Autodesk Inventor part; units mm, degrees
ref_plane "Plan YZ" through (0, 0, 0) normal (1, 0, 0) x (0, 1, 0)
ref_plane "Plan XZ" through (0, 0, 0) normal (0, 1, 0) x (-1, 0, 0)
ref_plane "Plan XY" through (0, 0, 0) normal (0, 0, 1) x (1, 0, 0)
sketch "Esquisse1" plane through (0, 0, 0) normal (0, 0, 1) x (1, 0, 0)
  line L0 (0, 0) -> (43.25, 0)
  line L1 (43.25, 0) -> (43.25, 42)
  line L2 (43.25, 42) -> (0, 42)
  line L3 (0, 42) -> (0, 0)
  dimension "d0" = 43.25
  dimension "d1" = 42
extrude "Extrusion1" add sketch "Esquisse1" along normal blind 1.6
sketch "Esquisse6" plane through (0, 0, 1.6) normal (0, 0, 1) x (1, 0, 0)
  line L0 (4.625, 38) -> (38.625, 38)
  line L1 (38.625, 38) -> (38.625, 4)
  line L2 (38.625, 4) -> (4.625, 4)
  line L3 (4.625, 4) -> (4.625, 38)
  line L4 (0, 27.3284) -> (4.625, 27.3284) construction
  line L5 (43.25, 21) -> (38.625, 21) construction
  line L6 (19.4191, 4) -> (19.4191, 0) construction
  line L7 (15.7943, 42) -> (15.7943, 38) construction
  line L8 (0, 0) -> (43.25, 0) construction
  line L9 (43.25, 42) -> (0, 42) construction
  line L10 (43.25, 0) -> (43.25, 42) construction
  line L11 (0, 42) -> (0, 0) construction
  dimension "d4" = 34
  dimension "d5" = 34
extrude "Extrusion2" add sketch "Esquisse6" along normal blind 1.9
sketch "Esquisse7" plane through (0, 0, 1.6) normal (0, 0, 1) x (1, 0, 0)
  line L0 (43.25, 0) -> (43.25, 42)
  line L1 (43.25, 42) -> (0, 42)
  point P0 (0, 0)
  point P1 (40.71, 39.46)
  dimension "d21" = 2.54
  dimension "d22" = 2.54
hole "Perçage1" at (40.71, 39.46, 1.6) direction (0, 0, -1) diameter 2.7 end through all
pattern_linear "Réseau rectangulaire1" count 2 spacing 36.9 along (0, -1, 0) count 2 spacing 38.1 along (-1, 0, 0) of "Perçage1"
sketch "Esquisse8" plane through (0, 0, 3.5) normal (0, 0, 1) x (1, 0, 0)
  line L0 (11.625, 24) -> (11.625, 19)
  line L1 (11.625, 19) -> (14.625, 19)
  line L2 (14.625, 19) -> (14.625, 20)
  line L3 (14.625, 20) -> (12.625, 20)
  line L4 (12.625, 20) -> (12.625, 24)
  line L5 (12.625, 24) -> (11.625, 24)
  line L6 (17.625, 24) -> (17.625, 19)
  line L7 (17.625, 19) -> (20.625, 19)
  line L8 (20.625, 19) -> (20.625, 20)
  line L9 (20.625, 20) -> (18.625, 20)
  line L10 (18.625, 20) -> (18.625, 21)
  line L11 (18.625, 21) -> (20.625, 21)
  line L12 (20.625, 21) -> (20.625, 22)
  line L13 (20.625, 22) -> (18.625, 22)
  line L14 (18.625, 22) -> (18.625, 23)
  line L15 (20.625, 23) -> (20.625, 24)
  line L16 (20.625, 24) -> (17.625, 24)
  line L17 (17.625, 24) -> (17.625, 24)
  line L18 (18.625, 23) -> (20.625, 23)
  line L19 (23.625, 19) -> (23.625, 24)
  line L20 (23.625, 24) -> (26.125, 24)
  line L21 (26.125, 24) -> (28.625, 21.5)
  line L22 (28.625, 21.5) -> (26.125, 19)
  line L23 (26.125, 19) -> (23.625, 19)
  line L24 (24.625, 20) -> (24.625, 23)
  line L25 (4.625, 38) -> (4.625, 4)
  line L26 (4.625, 4) -> (38.625, 4)
  line L27 (24.625, 20) -> (26.125, 20)
  line L28 (26.125, 20) -> (27.625, 21.5)
  line L29 (24.625, 23) -> (26.125, 23)
  line L30 (26.125, 23) -> (27.625, 21.5)
  point P0 (0, 0)
  dimension "d23" = 5
  dimension "d24" = 4
  dimension "d25" = 1
  dimension "d26" = 7
  dimension "d27" = 3
  dimension "d28" = 3
  dimension "d29" = 3
  dimension "d30" = 3
  dimension "d31" = 15
  dimension "d32" = 5
  dimension "d33" = 1
  dimension "d34" = 1
  dimension "d35" = 1
  dimension "d36" = 1
  dimension "d37" = 2
  dimension "d38" = 1
  dimension "d39" = 1
  dimension "d40" = 1
  dimension "d41" = 45
  dimension "d42" = 45
  dimension "d43" = 1
  dimension "d45" = 5
extrude "Extrusion3" cut sketch "Esquisse8" against normal blind 1
fillet "Congé1" radius 2 4 edges at (0, 42, 0.8) (43.25, 42, 0.8) (43.25, 0, 0.8) (0, 0, 0.8)
properties part number "P1704_014_Display" material "."
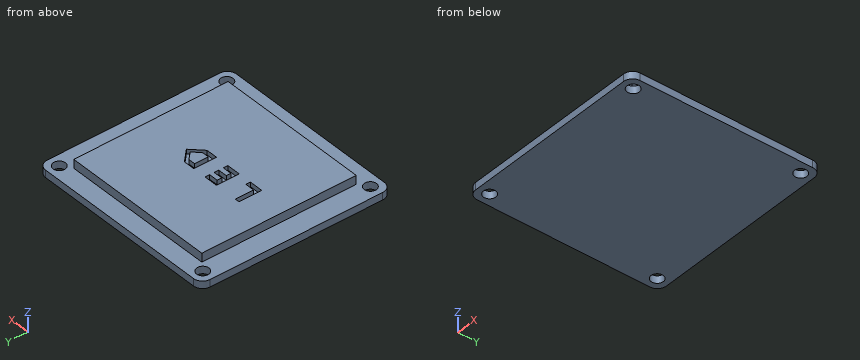
Source: CAD feature listing. Evaluate the final solid. Frame: model axes, mm. Round coordinates to 2 decimals unless told otherwise and drop trailing zeros. Order: outer loops, then holes, each group sorted by start corner. A loop starts at its lowest first (then second) coordinate and runs counter-clockwise, first axis right, second up. Notation, with made-up numbers: (0.5, 52.25) -> (32.5, 52.25) arc R16 cw to (32.5, 80.25) -> close; hole circle Ø1 at (86, 85.5). An arc over 180 degrees is marked (long way). One line per item, written item: value. Start each with the question number.
Q1. Material intervals for probe 1 along Y at (x, z) = (40.71, 1.05); probe 2 along X at (y, z) = (39.46, 1.25); probe 3 along Y at (x, z) = (18, 3.3), sorted ascending.
Q2. Pin query (flat end, axial travel): pin 1 (1.1 mm diameter, centred on x = 12, z = 3, fed in from -Y); pin 2 (1.1 mm diameter, centred on x = 19.5, z = 3, fed in from +Y); pin 3 (2.5 mm diameter, centred on x = 40.71, y = 2.56, fed in from -Z); pin 4 (1.1 mm diameter, centred on y = 21.5, z = 3, fed in from -X) (3 decimals). Return the tip coordinate at first contact, or that it passes through.
Q3. Section query C-C (x = 8). Return the cut outline in (y, z).
Q4. Section query B-B (y = 39.46). Return the cut outline in (x, z), plus the area to 3 significant figures.
Q5. Section query A-A (x = 2.61). Return the cut outline in (y, z), plus the area to 3 significant figures.
Q6. Section query D-D (y = 32.5). Return the cut outline in (x, z) (3 decimals), plus the area to 3 significant figures.
Findings below:
1. probe 1: 0 to 1.21, 3.91 to 38.11, 40.81 to 42
1. probe 2: 0 to 1.26, 3.96 to 39.36, 42.06 to 43.25
1. probe 3: 4 to 19, 24 to 38
2. pin 1: y = 4
2. pin 2: y = 38
2. pin 3: through
2. pin 4: x = 4.625
3. outline: (0, 0) -> (42, 0) -> (42, 1.6) -> (38, 1.6) -> (38, 3.5) -> (4, 3.5) -> (4, 1.6) -> (0, 1.6) -> close
4. outline: (0, 0) -> (1.26, 0) -> (1.26, 1.6) -> (0, 1.6) -> close; (3.96, 0) -> (39.36, 0) -> (39.36, 1.6) -> (3.96, 1.6) -> close; (42.06, 0) -> (43.25, 0) -> (43.25, 1.6) -> (42.06, 1.6) -> close
4. area: 60.6 mm²
5. outline: (0, 0) -> (1.21, 0) -> (1.21, 1.6) -> (0, 1.6) -> close; (3.91, 0) -> (38.11, 0) -> (38.11, 1.6) -> (3.91, 1.6) -> close; (40.81, 0) -> (42, 0) -> (42, 1.6) -> (40.81, 1.6) -> close
5. area: 58.6 mm²
6. outline: (0, 0) -> (43.25, 0) -> (43.25, 1.6) -> (38.625, 1.6) -> (38.625, 3.5) -> (4.625, 3.5) -> (4.625, 1.6) -> (0, 1.6) -> close
6. area: 134 mm²
